For this review, take the finished solid that the model builds, in its own axes (mm). Give positions to 0.01 mm unless a question says otherwise; leave off trailing zeros. Write each loop counter-clockwise with the first axis right and the second up, starting at its lowest first coordinate (ties: lowest second). Pieces come first, ordered by that corner, then holes. Notation, with made-up numbers: M -37,38 L 16,38 A7 ccw 16,49 Z; hole C -33.5,86.5 d10. An arc over 180 degrees is marked long. One line per item, written item: value. Start each with the question number.
Item 1: Clearance check with a flat-ended pin moving along its axis: pin 1 Ø1.5 at (x, y) = (1, 30.5) entering from -Z. State where the tip first meets the part, or that it passes through.
Item 2: To check wall thickness, follow probe 1 along Y at (x, z) = (-3.25, 5.5); probe 2 along X at (y, z) = (77.5, 5.25); probe 3 along X at (y, z) = (54.5, 3.5). State the ranges of each line that lie inside material, in increasing order.
Item 3: Consider section A-A, the plane y = 76. Write out the cut boundary in (x, z).
Item 4: Consider section B-B, the plane z = 1.25. Give the number of separate pieces and of enclosed holes in the cut face, and give its area (3 significant figures).
Item 5: Consider section D-D, the plane y = 50.5. Write out the cut boundary in (x, z), and give its area (3 significant figures).
```python
from build123d import *

# Parameters (mm, degrees)
SKETCH1_R           = 2.1
BOSS_EXTRUDE1_DEPTH = 6.35
SKETCH2_W           = 18.204542204
SKETCH2_H           = 91.842735445
CUT_EXTRUDE1_DEPTH  = 81.407229153
FILLET2_R           = 2


with BuildPart() as part:
    # Sketch1 → Boss-Extrude1 (new body)
    with BuildSketch(Plane.XY):
        with BuildLine():
            Line((3, -80), (-3, -80))
            ThreePointArc((-3, -80), (-4.414213562, -79.414213562), (-5, -78))
            Line((-5, -78), (-5, 78))
            ThreePointArc((-5, 78), (-4.414213562, 79.414213562), (-3, 80))
            Line((-3, 80), (3, 80))
            ThreePointArc((3, 80), (4.414213562, 79.414213562), (5, 78))
            Line((5, 78), (5, -78))
            ThreePointArc((5, -78), (4.414213562, -79.414213562), (3, -80))
        make_face()
        with Locations((0, 76)):
            Circle(SKETCH1_R, mode=Mode.SUBTRACT)
        with Locations((0, 69.391304348)):
            Circle(SKETCH1_R, mode=Mode.SUBTRACT)
        with Locations((0, 62.782608696)):
            Circle(SKETCH1_R, mode=Mode.SUBTRACT)
        with Locations((0, 56.173913043)):
            Circle(SKETCH1_R, mode=Mode.SUBTRACT)
        with Locations((0, 49.565217391)):
            Circle(SKETCH1_R, mode=Mode.SUBTRACT)
        with Locations((0, 42.956521739)):
            Circle(SKETCH1_R, mode=Mode.SUBTRACT)
        with Locations((0, 36.347826087)):
            Circle(SKETCH1_R, mode=Mode.SUBTRACT)
        with Locations((0, 29.739130435)):
            Circle(SKETCH1_R, mode=Mode.SUBTRACT)
        with Locations((0, 23.130434783)):
            Circle(SKETCH1_R, mode=Mode.SUBTRACT)
        with Locations((0, 16.52173913)):
            Circle(SKETCH1_R, mode=Mode.SUBTRACT)
        with Locations((0, 9.913043478)):
            Circle(SKETCH1_R, mode=Mode.SUBTRACT)
        with Locations((0, 3.304347826)):
            Circle(SKETCH1_R, mode=Mode.SUBTRACT)
        with Locations((0, -3.304347826)):
            Circle(SKETCH1_R, mode=Mode.SUBTRACT)
        with Locations((0, -9.913043478)):
            Circle(SKETCH1_R, mode=Mode.SUBTRACT)
        with Locations((0, -16.52173913)):
            Circle(SKETCH1_R, mode=Mode.SUBTRACT)
        with Locations((0, -23.130434783)):
            Circle(SKETCH1_R, mode=Mode.SUBTRACT)
        with Locations((0, -29.739130435)):
            Circle(SKETCH1_R, mode=Mode.SUBTRACT)
        with Locations((0, -36.347826087)):
            Circle(SKETCH1_R, mode=Mode.SUBTRACT)
        with Locations((0, -42.956521739)):
            Circle(SKETCH1_R, mode=Mode.SUBTRACT)
        with Locations((0, -49.565217391)):
            Circle(SKETCH1_R, mode=Mode.SUBTRACT)
        with Locations((0, -56.173913043)):
            Circle(SKETCH1_R, mode=Mode.SUBTRACT)
        with Locations((0, -62.782608696)):
            Circle(SKETCH1_R, mode=Mode.SUBTRACT)
        with Locations((0, -69.391304348)):
            Circle(SKETCH1_R, mode=Mode.SUBTRACT)
        with Locations((0, -76)):
            Circle(SKETCH1_R, mode=Mode.SUBTRACT)
    extrude(amount=BOSS_EXTRUDE1_DEPTH)

    # Sketch2 → Cut-Extrude1 (cut, through all)
    with BuildSketch(Plane(origin=(0, 0, 0), x_dir=(-1, 0, 0), z_dir=(0, 0, -1))):
        with Locations((-0.246007327, -39.312672071)):
            Rectangle(SKETCH2_W, SKETCH2_H)
    extrude(amount=-CUT_EXTRUDE1_DEPTH, mode=Mode.SUBTRACT)

    # Fillet2
    fillet2_edges = [part.edges().sort_by_distance(p)[0] for p in [
        (-5, 6.608695652, 3.175),
        (5, 6.608695652, 3.175),
    ]]
    fillet(fillet2_edges, radius=FILLET2_R)


solid = part.part
```
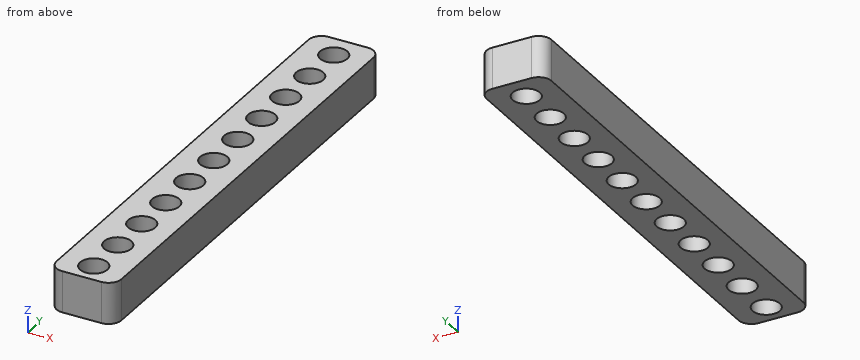
Model answer:
1. pin 1: passes through
2. probe 1: y = 6.62 to 79.98
2. probe 2: x = -5 to -1.47, 1.47 to 5
2. probe 3: x = -5 to -1.27, 1.27 to 5
3. outline: M -5,0 L -2.1,0 L -2.1,6.35 L -5,6.35 Z; M 2.1,0 L 5,0 L 5,6.35 L 2.1,6.35 Z
4. separate pieces: 1
4. enclosed holes: 11
4. area: 578 mm2
5. outline: M -5,0 L -1.88,0 L -1.88,6.35 L -5,6.35 Z; M 1.88,0 L 5,0 L 5,6.35 L 1.88,6.35 Z
5. area: 39.6 mm2
